Source: CAD feature listing. Evaluate the final solid. Frame: model axes, mm. Give positions to 0.01 mm unless a question says otherwise; leave off trailing zeros. Loops run counter-clockwise (first coordinate to the right, second up) from the corner with the lowest first, then second, coordinate; pieces in that order, holes last. Notation, with made-up numbers: M 73.5,38 L 117.5,38 A27 ccw 117.5,71 Z; hole C 57,-1 d1. An arc over 180 degrees is marked long. Answer in a Markdown table with one row per item.
Autodesk Inventor part; units mm, degrees
ref_plane "YZ Plane" through (0, 0, 0) normal (1, 0, 0) x (0, 1, 0)
ref_plane "XZ Plane" through (0, 0, 0) normal (0, 1, 0) x (-1, 0, 0)
ref_plane "XY Plane" through (0, 0, 0) normal (0, 0, 1) x (1, 0, 0)
sketch "Sketch1" plane through (0, 0, 0) normal (0, 0, 1) x (1, 0, 0)
  line L0 (0, 0) -> (184.15, 0)
  line L1 (84.0906, 44.45) -> (76.2, 32.0643)
  line L2 (76.2, 32.0643) -> (3.175, 15.875)
  line L3 (3.175, 15.875) -> (0, 0)
  circle A0 centre (0, 0) radius 190.5 construction
  line L4 (0, 0) -> (0, 190.5) construction
  line L5 (184.15, 0) -> (184.15, 25.4)
  line L6 (184.15, 25.4) -> (84.0906, 44.45)
  circle A1 centre (95.25, 12.7) radius 12
  dimension "d3" = 381
  dimension "d0" = 184.15
  dimension "d1" = 3.175
  dimension "d2" = 15.875
  dimension "d4" = 12.5
  dimension "d5" = 76.2
  dimension "d6" = 44.45
  dimension "d12" = 135
  dimension "d13" = 25.4
  dimension "d15" = 24
  dimension "d16" = 88.9
  dimension "d17" = 12.7
extrude "Extrusion1" add sketch "Sketch1" along normal blind 6.35 contours L3 L2 L1 L6 L5 L0 | A1
properties part number "Side_Blocker" material "UHMW, White"
1) Material intervals for L1, parallel to Y at x = 71, z = 2; L2, parallel to Y at x = 20, z = 1.5; L3, parallel to X at y = 8.5, z = 1, sorted ascending.
Reply:
| item | result |
|---|---|
| L1 | y = 0 to 30.91 |
| L2 | y = 0 to 19.61 |
| L3 | x = 1.7 to 184.15 |
2) Section A-A, the plane z = 3.75. Return loops of the section in (x, y) (3 decimals), then the cut area to 3 significant figures.
Reply:
| item | result |
|---|---|
| outline | M 0,0 L 184.15,0 L 184.15,25.4 L 84.091,44.45 L 76.2,32.064 L 3.175,15.875 Z |
| area | 5,570 mm² |
3) Pin query (flat end, axial travel): pin 1 Ø1.5 at (x, z) = (131.5, 3.5) entering from +Y. Return the tip coordinate at first contact, or that it passes through.
Reply:
| item | result |
|---|---|
| pin 1 | stops at y = 35.57 |
4) Section C-C, the plane y = 41. Return loops of the section in (x, z).
Reply:
| item | result |
|---|---|
| outline | M 81.89,0 L 102.21,0 L 102.21,6.35 L 81.89,6.35 Z |
5) Section B-B, the plane x = 48.5. Return loops of the section in (y, z).
Reply:
| item | result |
|---|---|
| outline | M 0,0 L 25.92,0 L 25.92,6.35 L 0,6.35 Z |
